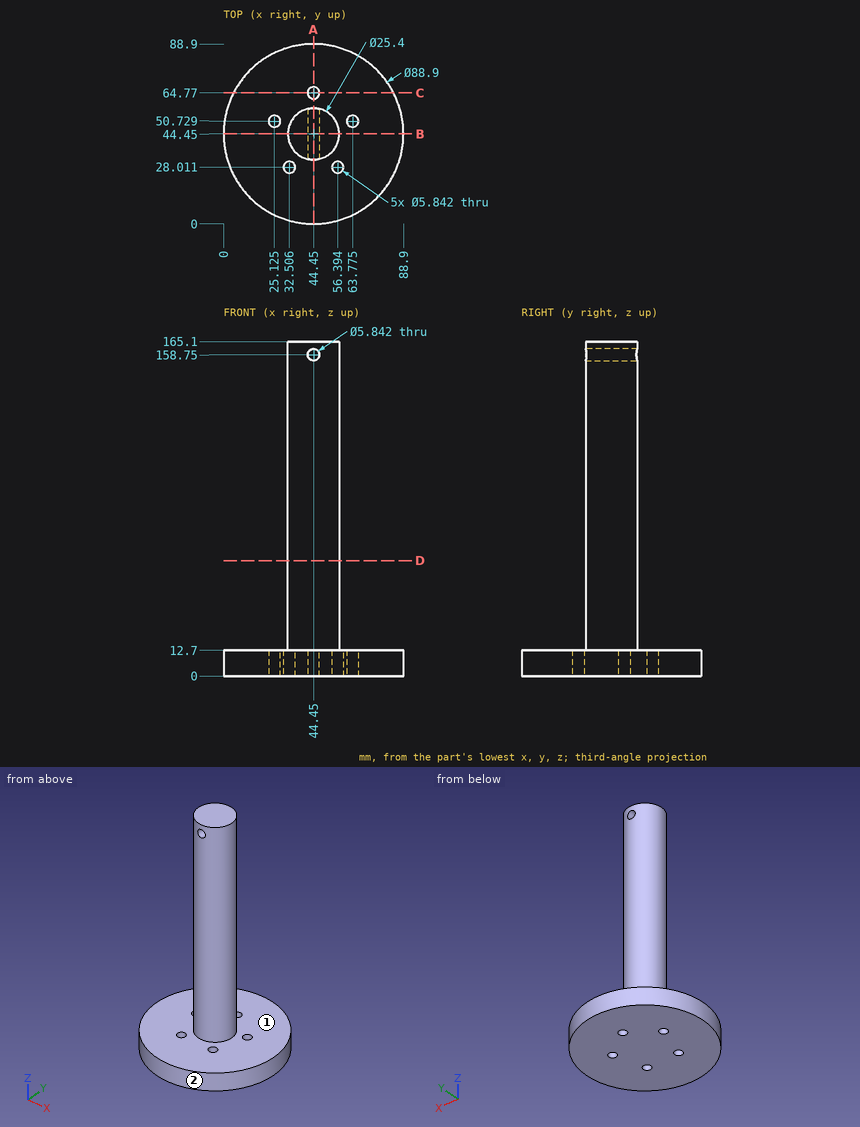
Can you work these out from the drawing? Everything is in mm from the part's minimum corner. A direction names the side the tool comes from. Give positions to 0.01 mm unless a question says otherwise; leave off trailing zeros. Order: outer loops, then holes, each group sorted by start corner. A loop starts at its lowest first (then second) coordinate and runs counter-clockwise, first axis right, second up.
1. Suppose I cut it at A-A (x = 44.45). List the corners of the cut face in (y, z) for me, plus the area to 3 significant figures.
2. I need wall thicknesses on L1, parallel to Z at x = 30.5, y = 65; L2, parallel to X at y = 39.25, z = 158.75 (1 decimal); L3, parallel to Y at x = 31.5, z = 11. Which ranges of each line are inside material? Lowest first, please.
3. Will these pins go through, and if not, where does the flat tip stop? P1, Ø1, axis at y = 47.5, z = 70.5, coming from the -X side; P2, Ø12, axis at x = 40.5, y = 27, coming from the +Z side; P3, Ø5, axis at x = 64, y = 46, coming from the +Z side; P4, Ø2, axis at y = 41.5, z = 141.5, coming from the +X side.
4. Suppose I cut it at D-D (z = 57). List the corners of the cut face in (x, y) for me, plus the area to 3 significant figures.
5. For the marked faces 1 and 2, which set-ups out of +Z, -Z, +X, -X, +Y, -Y let a thin tool reach every point of the face, with its end or its side?
6. Suppose I cut it at C-C (y = 64.77). List the corners of the cut face in (x, z) for me, plus the area to 3 significant figures.
7. Suppose I cut it at B-B (y = 44.45). List the corners of the cut face in (x, z) for me, plus the area to 3 significant figures.
Solved:
1. outline: (0, 0) - (61.85, 0) - (61.85, 12.7) - (57.15, 12.7) - (57.15, 155.83) - (31.75, 155.83) - (31.75, 12.7) - (0, 12.7) - close; (31.75, 161.67) - (57.15, 161.67) - (57.15, 165.1) - (31.75, 165.1) - close; (67.69, 0) - (88.9, 0) - (88.9, 12.7) - (67.69, 12.7) - close
1. area: 4,780 mm2
2. L1: z = 0 to 12.7
2. L2: x = 32.9 to 41.5, 47.4 to 56
2. L3: y = 1.93 to 25.27, 30.75 to 86.97
3. P1: stops at x = 32.01
3. P2: stops at z = 165.1
3. P3: stops at z = 12.7
3. P4: stops at x = 57
4. outline: circle Ø25.4 at (44.45, 44.45)
4. area: 507 mm2
5. face 1: +Z
5. face 2: +Z, -Z
6. outline: (4.92, 0) - (41.53, 0) - (41.53, 12.7) - (4.92, 12.7) - close; (47.37, 0) - (83.98, 0) - (83.98, 12.7) - (47.37, 12.7) - close
6. area: 930 mm2
7. outline: (0, 0) - (88.9, 0) - (88.9, 12.7) - (57.15, 12.7) - (57.15, 165.1) - (31.75, 165.1) - (31.75, 12.7) - (0, 12.7) - close; hole circle Ø5.84 at (44.45, 158.75)
7. area: 4,970 mm2
